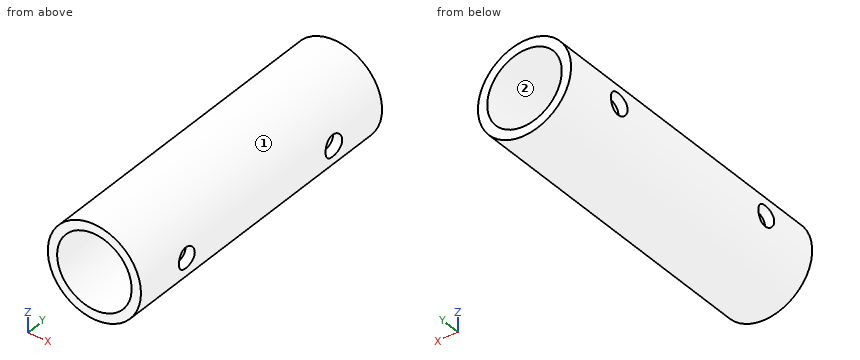
from build123d import *

# Parameters (mm, degrees)
F0_R     = 19.05
F1_DEPTH = 127
F2_R     = 15.24
F3_DEPTH = 127
F4_R     = 4.169678
F4_R_2   = 4.387646
F5_DEPTH = 50.8
F6_DEPTH = 25.4


with BuildPart() as f1:
    # F0 (on Front) → F1 (new body)
    with BuildSketch(Plane.XZ):
        Circle(F0_R)
    extrude(amount=F1_DEPTH)

    # F2 (on face) → F3 (cut)
    with BuildSketch(Plane(origin=(0, 0, 0), x_dir=(-1, 0, 0), z_dir=(0, 1, 0))):
        Circle(F2_R)
    extrude(amount=-F3_DEPTH, mode=Mode.SUBTRACT)

    # F4 (on Right) → F5 (cut)
    with BuildSketch(Plane.YZ):
        with Locations((-102.829032, 0)):
            Circle(F4_R)
        with Locations((-25.400002, 0)):
            Circle(F4_R_2)
    extrude(amount=-F5_DEPTH, mode=Mode.SUBTRACT)

    # F4 (on Right) → F6 (cut)
    with BuildSketch(Plane.YZ):
        with Locations((-102.829032, 0)):
            Circle(F4_R)
        with Locations((-25.400002, 0)):
            Circle(F4_R_2)
    extrude(amount=F6_DEPTH, mode=Mode.SUBTRACT)


solid = f1.part
Work out the finished part from the listing and answer in its coordinate system (mm). Face numbers are marked on the shaded views. Coordinates: 2 decimals unless noted, no trailing zeros. Write each loop counter-clockwise with the first axis right and the second up, starting at its lowest first coordinate (ties: lowest second). Pieces come first, ordered by that corner, then holes. Notation, with made-up numbers: (49.25, 88.25) - (95.25, 88.25) arc R16 cw to (95.25, 102.25) - close; hole circle Ø2 at (64, -9.75). An arc over 180 degrees is marked (long way). One line per question, with ' | ' between items.
1) The mould has two halves that part along Z. Classify the marked faces 1 and 2: +Z half, -Z half, draft (parallel to the pull), parting line (faces both ways), or undercut.
Checks:
face 1: parting line | face 2: undercut
2) Find section B-B, the plane z = 0. Determine the outline of the cut face in (x, y).
Checks:
outline: (-19.05, -127) - (-15.24, -127) - (-15.24, -107) - (-19.05, -107) - close; (-19.05, -98.66) - (-15.24, -98.66) - (-15.24, -29.79) - (-19.05, -29.79) - close; (-19.05, -21.01) - (-15.24, -21.01) - (-15.24, 0) - (-19.05, 0) - close; (15.24, -127) - (19.05, -127) - (19.05, -107) - (15.24, -107) - close; (15.24, -98.66) - (19.05, -98.66) - (19.05, -29.79) - (15.24, -29.79) - close; (15.24, -21.01) - (19.05, -21.01) - (19.05, 0) - (15.24, 0) - close
3) Find section A-A, the plane x = 0. Determine the outline of the cut face in (y, z).
Checks:
outline: (-127, -19.05) - (0, -19.05) - (0, -15.24) - (-127, -15.24) - close; (-127, 15.24) - (0, 15.24) - (0, 19.05) - (-127, 19.05) - close
4) Find section C-C, the plane y = -101.5. Determine the outline of the cut face in (x, z).
Checks:
outline: (-18.64, -3.95) arc R19.05 ccw to (18.64, -3.95) - (14.72, -3.95) arc R15.24 cw to (-14.72, -3.95) - close; (-18.64, 3.95) - (-14.72, 3.95) arc R15.24 cw to (14.72, 3.95) - (18.64, 3.95) arc R19.05 ccw to start
5) Find section D-D, the plane y = -38.5. Determine the outline of the cut face in (x, z).
Checks:
outline: circle Ø38.1 at (0, 0); hole circle Ø30.48 at (0, 0)
6) Consider probe 1 along Y at (x, z) = (16.4, 0); probe 2 along Z at (x, y) = (0, -62); probe 3 along Z at (x, y) = (13.5, -118). Determine where each line is inside the solid, lowest interval first. Write a range as [from, to].
Checks:
probe 1: [-127, -107], [-98.66, -29.79], [-21.01, 0] | probe 2: [-19.05, -15.24], [15.24, 19.05] | probe 3: [-13.44, -7.07], [7.07, 13.44]
7) Flat-ended cylindrical pins translate along their axes: P1, Ø3, axis at y = -109.5, z = 13.5, coming from the +X side; P2, Ø6.5, axis at y = -102.83, z = 0, coming from the -X side; P3, Ø8, axis at x = -14, y = -95, coming from the +Z side; P4, Ø12, axis at x = -6.5, y = -40, coming from the -Z side. Find the tip coordinate at first contact, or state that the pin passes through.
Checks:
P1: x = 14.8 | P2: through | P3: z = 16.21 | P4: z = -19.04
